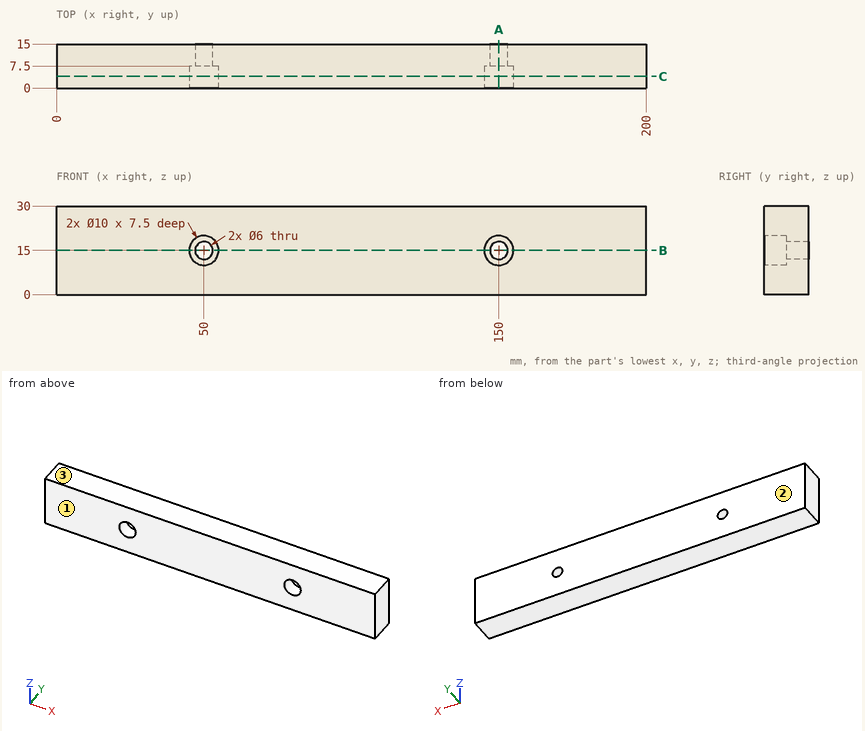
Design review of the part shown in the three views and the two pictorial views. Dimensions are in mm from the part's minimum x, y and z. Round coordinates to 2 decimals unless told otherwise and drop trailing zeros. Loops run counter-clockwise (first coordinate to the right, second up) from the corner with the lowest first, then second, coordinate; pieces in that order, holes last. Notation, with made-up numbers: M 71.5,49 L 130.5,49 A26 cw 130.5,81 Z; hole C 84.25,22.25 d5. An arc over 180 degrees is marked long. Put each result on its own line as item: value.
Q1. Consider section B-B, the plane z = 15. Give the boundary of the cut face in (x, y).
Result set:
outline: M 0,0 L 45,0 L 45,7.5 L 47,7.5 L 47,15 L 0,15 Z; M 53,7.5 L 55,7.5 L 55,0 L 145,0 L 145,7.5 L 147,7.5 L 147,15 L 53,15 Z; M 153,7.5 L 155,7.5 L 155,0 L 200,0 L 200,15 L 153,15 Z
Q2. For pin 1 (7 mm diameter, centred on x = 50, z = 15, fed in from -Y), flat-tipped, find the tip position at first contact; note if it passes through.
Result set:
pin 1: stops at y = 7.5
Q3. Mouldability with a two-part tool opening along Y and no side actions: class the marked faces 1, 2 and 3 as released by +Y, released by -Y, zero draft, split by the parting line, or undercut.
Result set:
face 1: released by -Y
face 2: released by +Y
face 3: zero draft
Q4. To check wall thickness, follow L1, parallel to Z at x = 50, y = 5.75; L2, parallel to X at y = 13, z = 16.5; L3, parallel to Z at x = 50, y = 13. State the ranges of each line that lie inside material, in increasing order.
Result set:
L1: z = 0 to 10, 20 to 30
L2: x = 0 to 47.4, 52.6 to 147.4, 152.6 to 200
L3: z = 0 to 12, 18 to 30
Q5. Consider section C-C, the plane y = 4. Give the boundary of the cut face in (x, z).
Result set:
outline: M 0,0 L 200,0 L 200,30 L 0,30 Z; hole C 50,15 d10; hole C 150,15 d10
Q6. Consider section A-A, the plane x = 150. Give the boundary of the cut face in (y, z), then the cut area to 3 significant figures.
Result set:
outline: M 0,0 L 15,0 L 15,12 L 7.5,12 L 7.5,10 L 0,10 Z; M 0,20 L 7.5,20 L 7.5,18 L 15,18 L 15,30 L 0,30 Z
area: 330 mm²
